from build123d import *

# Parameters (mm, degrees)
F0_W      = 42
F0_H      = 42
F1_DEPTH  = 40
F2_R      = 1.5
F3_DEPTH  = 4.5
F5_DEPTH  = 40.001
F6_R      = 11
F7_DEPTH  = 2
F8_R      = 2.5
F9_DEPTH  = 21
F11_DEPTH = 14
F12_W     = 12
F12_H     = 12
F13_DEPTH = 4
F14_W     = 1.5
F14_H     = 1
F15_DEPTH = 20


with BuildPart() as f1:
    # F0 (on Top) → F1 (new body)
    with BuildSketch(Plane.XY):
        Rectangle(F0_W, F0_H)
    extrude(amount=F1_DEPTH)

    # F2 (on face) → F3 (cut)
    with BuildSketch(Plane.XY.offset(40)):
        with Locations((15.5, 15.5)):
            Circle(F2_R)
        with Locations((15.5, -15.5)):
            Circle(F2_R)
        with Locations((-15.5, -15.5)):
            Circle(F2_R)
        with Locations((-15.5, 15.5)):
            Circle(F2_R)
    extrude(amount=-F3_DEPTH, mode=Mode.SUBTRACT)

    # F4 (on face) → F5 (cut, through all)
    with BuildSketch(Plane.XY.offset(40)):
        Polygon((17, 21), (21, 17), (21, 21), align=None)
        Polygon((17, -21), (21, -21), (21, -17), align=None)
        Polygon((-17, -21), (-21, -17), (-21, -21), align=None)
        Polygon((-17, 21), (-21, 21), (-21, 17), align=None)
    extrude(amount=-F5_DEPTH, mode=Mode.SUBTRACT)

    # F6 (on face) → F7 (join)
    with BuildSketch(Plane.XY.offset(40)):
        Circle(F6_R)
    extrude(amount=F7_DEPTH)

    # F8 (on face) → F9 (join)
    with BuildSketch(Plane.XY.offset(42)):
        Circle(F8_R)
    extrude(amount=F9_DEPTH)

    # F10 (on face) → F11 (cut)
    with BuildSketch(Plane.XY.offset(63)):
        with BuildLine():
            Line((-1.5, 2), (1.5, 2))
            ThreePointArc((1.5, 2), (0, 2.5), (-1.5, 2))
        make_face()
    extrude(amount=-F11_DEPTH, mode=Mode.SUBTRACT)

    # F12 (on face) → F13 (cut)
    with BuildSketch(Plane.XZ.offset(21)):
        with Locations((0, 9)):
            Rectangle(F12_W, F12_H)
    extrude(amount=-F13_DEPTH, mode=Mode.SUBTRACT)

    # F14 (on face) → F15 (join)
    with BuildSketch(Plane.XZ.offset(17)):
        with Locations((-3.9375, 9)):
            Rectangle(F14_W, F14_H)
        with Locations((-1.3125, 9)):
            Rectangle(F14_W, F14_H)
        with Locations((1.3125, 9)):
            Rectangle(F14_W, F14_H)
        with Locations((3.9375, 9)):
            Rectangle(F14_W, F14_H)
    extrude(amount=F15_DEPTH)


solid = f1.part
Input: part model. Units: mm. Frame: model coordinates. A direction names the side the tool comes from. Round coordinates to 2 decimals unless told otherwise and drop trailing zeros. Order: outer loops, then holes, each group sorted by start corner. A loop starts at its lowest first (then second) coordinate and runs counter-clockwise, first axis right, second up. Notation, with made-up numbers: (64.25, 64.25) - (77.25, 64.25) arc R14 ccw to (77.25, 83.25) - close; hole circle Ø4 at (-24.75, 32.25). An arc over 180 degrees is marked (long way). Use a Markdown table: item, result.
1. Access query for faces 1 (the face through (14, -15.43, 37.78)), 2 (the face through (6, -19, 9)), 3 (the face through (0, 2, 56)). Directions: +Z, -Z, +X, -X, +Y, -Y. A direction counts if a zero-diameter tool reaches every point of the face in a straight line with its end or side. Return the directions, or none.
Evaluation:
| item | result |
|---|---|
| face 1 | +Z |
| face 2 | -Y |
| face 3 | +Z, +X, -X, +Y |
2. Material intervals for probe 1 along Y at (x, z) = (-15.5, 38.25); probe 2 along Y at (x, z) = (15, 37), sorted ascending.
Evaluation:
| item | result |
|---|---|
| probe 1 | -21 to -17, -14 to 14, 17 to 21 |
| probe 2 | -21 to -16.91, -14.09 to 14.09, 16.91 to 21 |
3. Section A-A on y = -25. Return the cut outline in (x, z), then the cut area to 3 significant figures.
Evaluation:
| item | result |
|---|---|
| outline | (-4.69, 8.5) - (-3.19, 8.5) - (-3.19, 9.5) - (-4.69, 9.5) - close; (-2.06, 8.5) - (-0.56, 8.5) - (-0.56, 9.5) - (-2.06, 9.5) - close; (0.56, 8.5) - (2.06, 8.5) - (2.06, 9.5) - (0.56, 9.5) - close; (3.19, 8.5) - (4.69, 8.5) - (4.69, 9.5) - (3.19, 9.5) - close |
| area | 6.00 mm^2 |
4. Section B-B on y = 0. Return the cut outline in (x, z).
Evaluation:
| item | result |
|---|---|
| outline | (-21, 0) - (21, 0) - (21, 40) - (11, 40) - (11, 42) - (2.5, 42) - (2.5, 63) - (-2.5, 63) - (-2.5, 42) - (-11, 42) - (-11, 40) - (-21, 40) - close |
5. Section C-C on z = 11.5. Return the cut outline in (x, y), then the cut area to 3 significant figures.
Evaluation:
| item | result |
|---|---|
| outline | (-21, -17) - (-17, -21) - (-6, -21) - (-6, -17) - (6, -17) - (6, -21) - (17, -21) - (21, -17) - (21, 17) - (17, 21) - (-17, 21) - (-21, 17) - close |
| area | 1,680 mm^2 |
6. Section D-D on x = -13. Return the cut outline in (y, z), then the cut area to 3 significant figures.
Evaluation:
| item | result |
|---|---|
| outline | (-21, 0) - (21, 0) - (21, 40) - (-21, 40) - close |
| area | 1,680 mm^2 |
7. Mould query, pull axis Z, two halves, no side actions, for faces 4 (the face through (-6, -19, 9)), 5 (the face through (-17, -15.43, 37.78)), 6 (the face through (15, 16, 35.5)). Classes: +Z half, -Z half, draft (parallel to the pull), parting line (faces both ways), or undercut.
Evaluation:
| item | result |
|---|---|
| face 4 | undercut |
| face 5 | draft |
| face 6 | +Z half |
8. First-contact query: pin 1 (1.5 mm diameter, centred on y = -21.5, z = 8, fed in from +X); pin 2 (3.5 mm diameter, centred on x = 0.5, z = 56.5, fed in from +Y); pin 3 (1.1 mm diameter, centred on y = -25.5, z = 9, fed in from +X). Flat tips, straight axial feed; report the tip coordinate or a pass-through.
Evaluation:
| item | result |
|---|---|
| pin 1 | x = 17.25 |
| pin 2 | y = 2 |
| pin 3 | x = 4.69 |
